Autodesk Inventor part; units mm, degrees
ref_plane "YZ Plane" through (0, 0, 0) normal (1, 0, 0) x (0, 1, 0)
ref_plane "XZ Plane" through (0, 0, 0) normal (0, 1, 0) x (-1, 0, 0)
ref_plane "XY Plane" through (0, 0, 0) normal (0, 0, 1) x (1, 0, 0)
sketch "Эскиз1" plane through (0, 0, 0) normal (0, 1, 0) x (-1, 0, 0)
  line L0 (-2.9, 6.425) -> (2.9, 6.425)
  line L1 (2.9, 6.425) -> (2.9, -6.425)
  line L2 (2.9, -6.425) -> (-2.9, -6.425)
  line L3 (-2.9, -6.425) -> (-2.9, 6.425)
  line L4 (-2.9, 6.425) -> (2.9, -6.425) construction
  line L5 (2.9, 6.425) -> (-2.9, -6.425) construction
  line L6 (-3, 6.35) -> (3, 6.35)
  line L7 (3, 6.35) -> (3, -6.35)
  line L8 (3, -6.35) -> (-3, -6.35)
  line L9 (-3, -6.35) -> (-3, 6.35)
  line L10 (-3, 6.35) -> (3, -6.35) construction
  line L11 (3, 6.35) -> (-3, -6.35) construction
  line L12 (3, 6.35) -> (4.3, 6.35)
  line L13 (4.3, 6.35) -> (4.3, -6.35)
  line L14 (4.3, -6.35) -> (3, -6.35)
  line L15 (3, -6.35) -> (3, 6.35)
  line L16 (-3, 6.35) -> (-4.3, 6.35)
  line L17 (-4.3, 6.35) -> (-4.3, -6.35)
  line L18 (-4.3, -6.35) -> (-3, -6.35)
  line L19 (-3, -6.35) -> (-3, 6.35)
  point P0 (0, 0)
  dimension "d0" = 5.8
  dimension "d1" = 12.85
  dimension "d2" = 6
  dimension "d3" = 12.7
  dimension "d4" = 1.3
  dimension "d5" = 1.3
extrude "Выдавливание1" add sketch "Эскиз1" along normal blind 8.1 contours L6 L1 L8 L3 | L3 L8 L9 L6 | L6 L7 L8 L1 | L9 L18 L17 L16 | L12 L13 L14 L7
sketch "Эскиз2" plane through (0, 8.1, 0) normal (0, 1, 0) x (1, 0, 0)
  line L0 (4.3, 6.35) -> (-4.3, 6.35)
  line L1 (3, -6.35) -> (-3, -6.35)
  line L2 (-3, -6.35) -> (-3, 6.35)
  line L3 (-3, 6.35) -> (3, 6.35)
  line L4 (3, 6.35) -> (3, -6.35)
  line L5 (3, -6.35) -> (-3, 6.35) construction
  line L6 (-3, -6.35) -> (3, 6.35) construction
  point P0 (0, 0)
  dimension "d8" = 6
extrude "Выдавливание2" cut sketch "Эскиз2" against normal blind 3.8
sketch "Эскиз3" plane through (0, 4.3, 0) normal (0, 1, 0) x (1, 0, 0)
  line L0 (3, 6.35) -> (3, -6.35)
  line L1 (-3, 6.35) -> (3, 6.35)
  line L2 (-3, -6.35) -> (-3, 6.35)
  line L3 (3, -6.35) -> (-3, -6.35)
  line L4 (3, -6.35) -> (1.7, -6.35)
  line L5 (-4.3, -6.35) -> (4.3, -6.35)
  line L6 (-3, -6.35) -> (-0.75, -6.35)
  line L7 (-0.75, -6.35) -> (-0.75, 6.35)
  line L8 (1.7, -6.35) -> (1.7, 6.35)
  line L9 (-3, 6.35) -> (3, 6.35)
  line L10 (-0.75, -6.35) -> (1.7, -6.35)
  line L11 (0.475, -6.35) -> (0.475, 6.35)
  line L12 (0.475, -5.08) -> (0.475, 0)
  line L13 (0.475, 0) -> (0.475, 5.08)
  line L14 (1.7, 0) -> (-0.75, 0)
  line L15 (-0.75, -0.675) -> (1.7, -0.675)
  line L16 (1.7, -0.675) -> (1.7, 0.675)
  line L17 (1.7, 0.675) -> (-0.75, 0.675)
  line L18 (-0.75, 0.675) -> (-0.75, -0.675)
  line L19 (-0.75, -0.675) -> (1.7, 0.675) construction
  line L20 (1.7, -0.675) -> (-0.75, 0.675) construction
  line L21 (-0.75, 4.405) -> (1.7, 4.405)
  line L22 (1.7, 4.405) -> (1.7, 5.755)
  line L23 (1.7, 5.755) -> (-0.75, 5.755)
  line L24 (-0.75, 5.755) -> (-0.75, 4.405)
  line L25 (-0.75, 4.405) -> (1.7, 5.755) construction
  line L26 (1.7, 4.405) -> (-0.75, 5.755) construction
  line L27 (-0.75, -5.755) -> (1.7, -5.755)
  line L28 (1.7, -5.755) -> (1.7, -4.405)
  line L29 (1.7, -4.405) -> (-0.75, -4.405)
  line L30 (-0.75, -4.405) -> (-0.75, -5.755)
  line L31 (-0.75, -5.755) -> (1.7, -4.405) construction
  line L32 (1.7, -5.755) -> (-0.75, -4.405) construction
  line L33 (-0.95, 0.875) -> (1.9, 0.875)
  line L34 (1.9, 0.875) -> (1.9, -0.875)
  line L35 (1.9, -0.875) -> (-0.95, -0.875)
  line L36 (-0.95, -0.875) -> (-0.95, 0.875)
  line L37 (1.9, 4.205) -> (-0.95, 4.205)
  line L38 (-0.95, 4.205) -> (-0.95, 5.955)
  line L39 (-0.95, 5.955) -> (1.9, 5.955)
  line L40 (1.9, 5.955) -> (1.9, 4.205)
  line L41 (-0.95, -4.205) -> (1.9, -4.205)
  line L42 (1.9, -4.205) -> (1.9, -5.955)
  line L43 (1.9, -5.955) -> (-0.95, -5.955)
  line L44 (-0.95, -5.955) -> (-0.95, -4.205)
  line L45 (-0.95, 5.955) -> (1.9, 5.955)
  line L46 (1.9, 5.955) -> (1.9, 4.205)
  line L47 (1.9, 4.205) -> (-0.95, 4.205)
  line L48 (-0.95, 4.205) -> (-0.95, 5.955)
  point P0 (0, 0)
  point P1 (-0.75, -4.205)
  point P2 (-0.75, -5.955)
  point P3 (-0.75, 4.205)
  point P4 (-0.75, 5.955)
  point P5 (-0.75, 5.955)
  dimension "d11" = 1.3
  dimension "d12" = 2.25
  dimension "d13" = 5.08
  dimension "d14" = 5.08
  dimension "d15" = 1.35
  dimension "d16" = 1.35
  dimension "d17" = 1.35
  dimension "d18" = 0.2
  dimension "d19" = 0.2
  dimension "d20" = 0.2
extrude "Выдавливание3" cut sketch "Эскиз3" against normal blind 4 contours L39 L40 L37 L8 | L8 L23 L11 L39 | L43 L11 L27 L8 | L8 L41 L42 L43 | L11 L23 L7 L39 | L8 L21 L11 L23 | L43 L7 L27 L11 | L27 L11 L29 L8 | L7 L37 L38 L39 | L11 L21 L7 L23 | L8 L37 L11 L21 | L27 L7 L29 L11 | L29 L11 L41 L8 | L11 L37 L7 L21 | L29 L7 L41 L11 | L33 L34 L35 L8 | L8 L17 L11 L33 | L35 L11 L15 L8 | L8 L14 L11 L17 | L11 L17 L7 L33 | L15 L11 L14 L8 | L35 L7 L15 L11 | L7 L35 L36 L33 | L11 L14 L7 L17 | L15 L7 L14 L11
sketch "Эскиз4" plane through (0, 0.3, 0) normal (0, 1, 0) x (1, 0, 0)
  line L0 (1.9, -5.955) -> (-0.75, -5.955)
  line L1 (-0.75, -5.955) -> (-0.75, -4.205)
  line L2 (-0.75, -4.205) -> (1.9, -4.205)
  line L3 (1.9, -4.205) -> (1.9, -5.955)
  line L4 (1.9, 5.955) -> (1.9, 4.205)
  line L5 (1.9, 4.205) -> (-0.95, 4.205)
  line L6 (-0.95, 4.205) -> (-0.95, 5.955)
  line L7 (-0.95, 5.955) -> (1.9, 5.955)
  line L8 (1.9, -0.875) -> (-0.95, -0.875)
  line L9 (-0.95, -0.875) -> (-0.95, 0.875)
  line L10 (-0.95, 0.875) -> (1.9, 0.875)
  line L11 (1.9, 0.875) -> (1.9, -0.875)
  line L12 (3, 6.35) -> (3, -6.35)
  line L13 (-3, 6.35) -> (3, 6.35)
  line L14 (-3, -6.35) -> (-3, 6.35)
  line L15 (3, -6.35) -> (-3, -6.35)
  line L16 (0, -0.875) -> (-0.4, -0.875)
  line L17 (-0.4, -0.875) -> (-0.4, 0.875)
  line L18 (-0.4, 0.875) -> (0, 0.875)
  line L19 (0, 0.875) -> (0, -0.875)
  line L20 (1.9, 4.205) -> (-0.95, 4.205)
  line L21 (0, 4.205) -> (-0.4, 4.205)
  line L22 (-0.4, 4.205) -> (-0.4, 5.955)
  line L23 (-0.4, 5.955) -> (0, 5.955)
  line L24 (0, 5.955) -> (0, 4.205)
  line L25 (1.9, -5.955) -> (-0.75, -5.955)
  line L26 (-0.75, -4.205) -> (1.9, -4.205)
  line L27 (0, -5.955) -> (-0.4, -5.955)
  line L28 (-0.4, -5.955) -> (-0.4, -4.205)
  line L29 (-0.4, -4.205) -> (0, -4.205)
  line L30 (0, -4.205) -> (0, -5.955)
  line L31 (3, -6.35) -> (-3, -6.35)
  line L32 (0, -6.35) -> (0, 6.35)
  line L33 (4.3, 6.35) -> (-4.3, 6.35)
  point P0 (0, 0)
  dimension "d23" = 0.4
extrude "Выдавливание4" cut sketch "Эскиз4" against normal blind 4 contours L0 L28 L2 L30 | L8 L17 L10 L19 | L5 L22 L7 L24
fillet "Сопряжение1" radius 1 4 edges at (4.3, 4.05, 6.35) (-4.3, 4.05, 6.35) (-4.3, 4.05, -6.35) (4.3, 4.05, -6.35)
properties part number "push-fit"
CAD build for the part. Positions are in the model's coordinates, mm. A direction names the side the tool comes from. Round coordinates to 2 decimals unless told otherwise and drop trailing zeros. Loops run counter-clockwise (first coordinate to the right, second up) from the corner with the lowest first, then second, coordinate; pieces in that order, holes last.
(1) Which spindle directions (+Z, -Z, +X, -X, +Y, -Y) get a long thin tool onto all of the face, cutting with end or side? Do faces 1 (the flat face through (1, 2, 4.205)), 2 (the flat face through (4.3, 4, 0)), 3 (the flat face through (-3, 6, 0)). Say none if no direction does.
(2) Drop a flat-ended pin along its axis: pin 1 (0.5 mm diameter, centred on x = 1, z = 5, fed in from +Y). Give the stop position or say it passes through.
(3) Wall check: line 1 along Z through (x, y) = (1, 0.5) (3 decimals); line 2 along X through (y, z) = (2.75, 4.25); line 3 along X through (y, z) = (4, -4.75). Give the ranges that are in metal, low to high.
(4) Two-plate mould, pull along X, no slides. Class faces 4 (the cylindrical face through (3.999, 4.107, 6.065)), 5 (the flat face through (1, 2, 5.955)), 6 (the flat face through (4, 8.1, 0)): +X half, -X half, draft (parallel to the pull), parting line (faces both ways), or undercut.
(5) Cut at C-C (z = -3). Give the cut face in (x, y), plus the area to 3 significant figures.
(6) Cut at A-A (y = 5.25). Give the cut face in (x, z), plus the area to 3 significant figures.
(7) Cut at B-B (z = -4.5). Give the cut face in (x, y).
(8) Cut at D-D (y = 2). Give the cut face in (x, z) (3 decimals).
Findings below:
1. face 1: +Y
1. face 2: +Z, -Z, +X, +Y, -Y
1. face 3: +Z, -Z, +Y
2. pin 1: stops at y = 0.3
3. line 1: z = -6.35 to -5.955, -4.205 to -0.875, 0.875 to 4.205, 5.955 to 6.35
3. line 2: x = -4.3 to -0.75, 1.9 to 4.3
3. line 3: x = -4.3 to -0.95, 1.9 to 4.3
4. face 4: +X half
4. face 5: undercut
4. face 6: draft
5. outline: (-4.3, 0) - (4.3, 0) - (4.3, 8.1) - (3, 8.1) - (3, 4.3) - (-3, 4.3) - (-3, 8.1) - (-4.3, 8.1) - close
5. area: 46.9 mm2
6. outline: (-4.3, -5.35) arc R1 ccw to (-3.3, -6.35) - (-3, -6.35) - (-3, 6.35) - (-3.3, 6.35) arc R1 ccw to (-4.3, 5.35) - close; (3, -6.35) - (3.3, -6.35) arc R1 ccw to (4.3, -5.35) - (4.3, 5.35) arc R1 ccw to (3.3, 6.35) - (3, 6.35) - close
6. area: 32.2 mm2
7. outline: (-4.3, 0) - (-0.4, 0) - (-0.4, 0.3) - (-0.95, 0.3) - (-0.95, 4.3) - (-3, 4.3) - (-3, 8.1) - (-4.3, 8.1) - close; (0, 0) - (4.3, 0) - (4.3, 8.1) - (3, 8.1) - (3, 4.3) - (1.9, 4.3) - (1.9, 0.3) - (0, 0.3) - close
8. outline: (-4.3, -5.35) arc R1 ccw to (-3.3, -6.35) - (3.3, -6.35) arc R1 ccw to (4.3, -5.35) - (4.3, 5.35) arc R1 ccw to (3.3, 6.35) - (-3.3, 6.35) arc R1 ccw to (-4.3, 5.35) - close; hole (-0.95, -5.955) - (1.9, -5.955) - (1.9, -4.205) - (-0.95, -4.205) - close; hole (-0.95, -0.875) - (1.9, -0.875) - (1.9, 0.875) - (-0.95, 0.875) - close; hole (-0.75, 4.205) - (1.9, 4.205) - (1.9, 5.955) - (-0.75, 5.955) - close
